The listing builds one solid part. Answer for the finished solid, in the listing's coordinates (mm). Coordinates: 2 decimals unless noted, no trailing zeros. Loops run counter-clockwise (first coordinate to the right, second up) from the corner with the lowest first, then second, coordinate; pieces in that order, holes last. Notation, with made-up numbers: (38.5, -14) - (86.5, -14) arc R21 cw to (86.5, -9) - close; hole circle Ø3 at (9, 78.5). An arc over 180 degrees is marked (long way). Write each question's results on one line, items separated by ' | '. Start each with the question number.
(1) Consider line 1 (Y direction, x = 95, z = 12); line 2 (Y direction, x = 0, z = 5.25); line 3 (X direction, y = 3, z = 10.5). Determine where each line is inside the solid, lowest interval first. Write a range as from..to.
(2) Find section A-A on x = -50. Determine the outline of the cut face in (y, z).
(3) Find section D-D on y = 0. Determine the outline of the cut face in (x, z).
(4) Given pin 1 Ø9 at (x, y) = (0, 0) entering from -Z; pin 2 Ø15 at (x, y) = (-95, -12.5) entering from +Z; pin 3 Ø17.5 at (x, y) = (58, 0.5) entering from +Z, each flat-ended and moving along its own axis, determine where each tip first touches the part or whether it passes through.
(5) Find section C-C on x = -95. Determine the outline of the cut face in (y, z), then the cut area to 3 significant figures.
(6) Find section B-B on z = 4. Determine the outline of the cut face in (x, y), then the cut area to 3 significant figures.
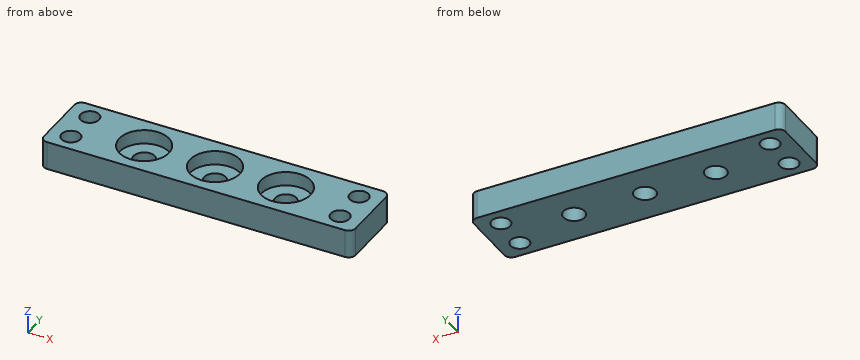
from build123d import *

# Parameters (mm, degrees)
F0_W     = 220
F0_H     = 50
F0_R     = 7.5
F1_DEPTH = 20
F2_D     = 13.2
F3_R     = 5
F4_R     = 17.5
F4_R_2   = 7.5
F5_DEPTH = 10


with BuildPart() as f1:
    # F0 (on Top) → F1 (new body)
    with BuildSketch(Plane.XY):
        Rectangle(F0_W, F0_H)
        with Locations((-50, 0)):
            Circle(F0_R, mode=Mode.SUBTRACT)
        Circle(F0_R, mode=Mode.SUBTRACT)
        with Locations((50, 0)):
            Circle(F0_R, mode=Mode.SUBTRACT)
    extrude(amount=F1_DEPTH)

    # F2 (through all)
    with Locations(Plane(origin=(0, 0, 0), x_dir=(1, 0, 0), z_dir=(0, 0, -1))):
        with Locations((-95, -12.5), (-95, 12.5), (95, -12.5), (95, 12.5)):
            Hole(F2_D / 2)

    # F3
    f3_edges = [f1.edges().sort_by_distance(p)[0] for p in [
        (-110, -25, 10),
        (110, -25, 10),
        (110, 25, 10),
        (-110, 25, 10),
    ]]
    fillet(f3_edges, radius=F3_R)

    # F4 (on face) → F5 (cut)
    with BuildSketch(Plane.XY.offset(20)):
        with Locations((-50, 0)):
            Circle(F4_R)
        with Locations((-50, 0)):
            Circle(F4_R_2, mode=Mode.SUBTRACT)
        with Locations((50, 0)):
            Circle(F4_R)
        with Locations((50, 0)):
            Circle(F4_R_2, mode=Mode.SUBTRACT)
        Circle(F4_R)
        Circle(F4_R_2, mode=Mode.SUBTRACT)
    extrude(amount=-F5_DEPTH, mode=Mode.SUBTRACT)


solid = f1.part
Values:
1) line 1: y = -25..-19.1, -5.9..5.9, 19.1..25 | line 2: y = -25..-7.5, 7.5..25 | line 3: x = -110..-67.24, -32.76..-17.24, 17.24..32.76, 67.24..110
2) outline: (-25, 0) - (-7.5, 0) - (-7.5, 10) - (-17.5, 10) - (-17.5, 20) - (-25, 20) - close; (7.5, 0) - (25, 0) - (25, 20) - (17.5, 20) - (17.5, 10) - (7.5, 10) - close
3) outline: (-110, 0) - (-57.5, 0) - (-57.5, 10) - (-67.5, 10) - (-67.5, 20) - (-110, 20) - close; (-42.5, 0) - (-7.5, 0) - (-7.5, 10) - (-17.5, 10) - (-17.5, 20) - (-32.5, 20) - (-32.5, 10) - (-42.5, 10) - close; (7.5, 0) - (42.5, 0) - (42.5, 10) - (32.5, 10) - (32.5, 20) - (17.5, 20) - (17.5, 10) - (7.5, 10) - close; (57.5, 0) - (110, 0) - (110, 20) - (67.5, 20) - (67.5, 10) - (57.5, 10) - close
4) pin 1: passes through | pin 2: stops at z = 20 | pin 3: stops at z = 10
5) outline: (-25, 0) - (-19.1, 0) - (-19.1, 20) - (-25, 20) - close; (-5.9, 0) - (5.9, 0) - (5.9, 20) - (-5.9, 20) - close; (19.1, 0) - (25, 0) - (25, 20) - (19.1, 20) - close | area: 472 mm²
6) outline: (-110, -20) arc R5 ccw to (-105, -25) - (105, -25) arc R5 ccw to (110, -20) - (110, 20) arc R5 ccw to (105, 25) - (-105, 25) arc R5 ccw to (-110, 20) - close; hole circle Ø13.2 at (-95, -12.5); hole circle Ø13.2 at (-95, 12.5); hole circle Ø15 at (-50, 0); hole circle Ø15 at (0, 0); hole circle Ø15 at (50, 0); hole circle Ø13.2 at (95, -12.5); hole circle Ø13.2 at (95, 12.5) | area: 9,900 mm²
